Can you work these out from the drawing? Everything is in mm from the part's minimum corner. A direction names the side the tool comes from. Round coordinates to 2 decimals unless told otherwise and drop trailing zeros. Write each loop counter-clockwise with the first axis right and the second up, starting at its lowest first coordinate (ties: lowest second). Pieces come first, ordered by that corner, then holes. Notation, with made-up numbers: M 64.25,53.5 L 107.25,53.5 A24 ccw 107.25,73.5 Z; hole C 63.25,82.5 d3. An arc over 180 degrees is marked long. Use a Markdown table: item, result. Add a question column.
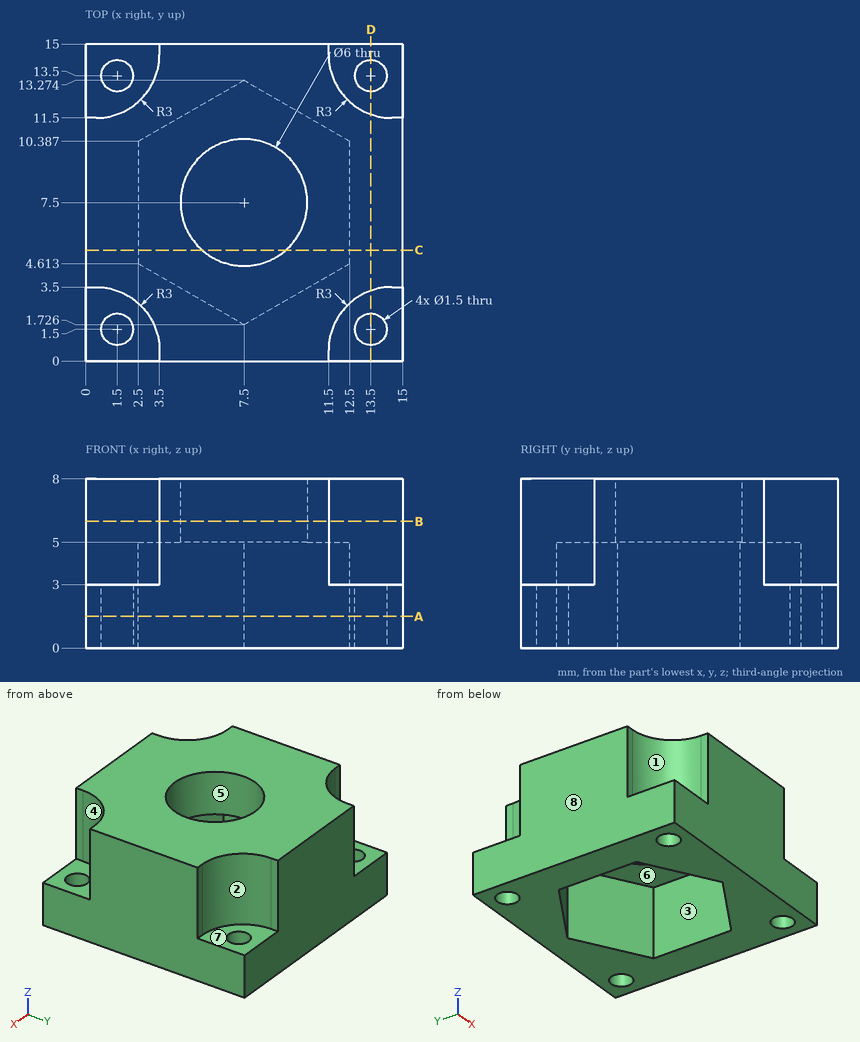
Item 1: If we mould it in two halves opening along X, with no side actions, what happens to the marked faces 1, 2 and 3? For each: +X half, -X half, draft (parallel to the pull), parting line (faces both ways), or undercut.
Item 2: Imagine slicing it at B-B on z = 6. List the corners of the cut face in (x, y) for me.
Item 3: On a 3-axis mill with a long thin cutter (end or side, diameter ignored), from which of +Z, -Z, +X, -X, +Y, -Y can I reach the whole of each face in a straight line? I mean the marked faces 4, 5, 6, 7 and 8. Say none if no direction works.
Item 4: Imagine slicing it at C-C on y = 5.25. List the corners of the cut face in (x, z) for me (1 decimal).
Item 5: For pin 1 Ø2.5 at (x, y) = (1.5, 13.5) entering from +Z; pin 2 Ø1.5 at (y, z) = (1.5, 6) entering from +X; pin 3 Ø1.5 at (x, y) = (11.5, 6.5) entering from -Z, each with a flat end and sliding along its axis, tell me the tip position at first contact or that it passes through.
Item 6: Imagine slicing it at A-A on z = 1.5. List the corners of the cut face in (x, y) for me, plus the area to 3 significant figures.
Item 7: Imagine slicing it at D-D on x = 13.5. List the corners of the cut face in (y, z) for me.
Item 8: I need wall thicknesses on probe 1 along Y at (x, z) = (1.5, 2.1); probe 2 along Y at (x, z) = (7.5, 7.3); probe 3 along X at (y, z) = (7.5, 1.25). Which ranges of each line are inside material? Lowest first, please. Write a range as from..to.
The answers:
| question | item | result |
|---|---|---|
| 1 | face 1 | -X half |
| 1 | face 2 | +X half |
| 1 | face 3 | undercut |
| 2 | outline | M 0,3.5 L 0.5,3.5 A3 cw 3.5,0.5 L 3.5,0 L 11.5,0 L 11.5,0.5 A3 cw 14.5,3.5 L 15,3.5 L 15,11.5 L 14.5,11.5 A3 cw 11.5,14.5 L 11.5,15 L 3.5,15 L 3.5,14.5 A3 cw 0.5,11.5 L 0,11.5 Z; hole C 7.5,7.5 d6 |
| 3 | face 4 | +Z, +X, -Y |
| 3 | face 5 | +Z, -Z |
| 3 | face 6 | -Z |
| 3 | face 7 | +Z, +X, +Y |
| 3 | face 8 | +Z, -Z, -X, +Y, -Y |
| 4 | outline | M 0,0 L 2.5,0 L 2.5,5 L 5.5,5 L 5.5,8 L 0,8 Z; M 9.5,5 L 12.5,5 L 12.5,0 L 15,0 L 15,8 L 9.5,8 Z |
| 5 | pin 1 | z = 3 |
| 5 | pin 2 | x = 12.06 |
| 5 | pin 3 | z = 5 |
| 6 | outline | M 0,0 L 15,0 L 15,15 L 0,15 Z; hole C 1.5,1.5 d1.5; hole C 1.5,13.5 d1.5; hole M 2.5,4.61 L 7.5,1.73 L 12.5,4.61 L 12.5,10.39 L 7.5,13.27 L 2.5,10.39 Z; hole C 13.5,1.5 d1.5; hole C 13.5,13.5 d1.5 |
| 6 | area | 131 mm² |
| 7 | outline | M 0,0 L 0.75,0 L 0.75,3 L 0,3 Z; M 2.25,0 L 12.75,0 L 12.75,3 L 11.67,3 L 11.67,8 L 3.33,8 L 3.33,3 L 2.25,3 Z; M 14.25,0 L 15,0 L 15,3 L 14.25,3 Z |
| 8 | probe 1 | 0..0.75, 2.25..12.75, 14.25..15 |
| 8 | probe 2 | 0..4.5, 10.5..15 |
| 8 | probe 3 | 0..2.5, 12.5..15 |
